Read the model definition and answer for the solid it produces. Units are mm, in the model's axes. A direction names the side the tool comes from. Coordinates: 2 decimals unless noted, no trailing zeros. Loops run counter-clockwise (first coordinate to the right, second up) from the corner with the lowest first, then second, coordinate; pieces in that order, holes last. Notation, with made-up numbers: M -32.5,1 L -12.5,1 A22 cw -12.5,21 Z; hole C 55.5,65 d4. An arc over 180 degrees is marked long. Use one line per item in the form item = value. Start each with the question number.
1. A tool of negligible diameter and unlimited length cuts with its end or side. For faces 4 (the flat face through (8.128, -19, 99)), 5 (the cylindrical face through (26.798, 52.192, 92.535)), from which of +Z, -Z, +X, -X, +Y, -Y can it reach the whole face along a straight path? Write none if from no direction.
2. The part is cut by section D-D (x = 4.5). Give the vertices of the cut face in (y, z), plus the area to 3 significant figures.
3. Find the intervals of material crossed by probe 1 along X at (y, z) = (-22, 98); probe 2 along Y at (x, z) = (21, 9); probe 3 along Z at (x, y) = (47, 33), in increasing order. Write a range as [from, to].
4. For a pull along X with two mould halves and no side action, classify faces 1 (the flat face through (46.228, -19, 99)), 2 (the flat face through (54.356, 10, 54)), 3 (the cylindrical face through (4.01, -15.1, 101.36)) as released by +X, released by -X, zero draft, split by the parting line, or undercut.
5. The part is cut by section A-A (x = 28.5). Give the vertices of the cut face in (y, z).
6. The part is cut by section B-B (z = 9). Give the vertices of the cut face in (x, y).
7. Flat-ended cylindrical pins translate along their axes: pin 1 (13 mm diameter, centred on y = -18, z = 102, fed in from -X); pin 2 (1 mm diameter, centred on x = 46, z = 40, fed in from +Y); pin 3 (12 mm diameter, centred on x = 44, y = 19, fed in from +Z); pin 4 (5 mm diameter, centred on x = 9.5, y = -18.5, fed in from +Z). Find the tip coordinate at first contact, or state that the pin passes through.
8. The part is cut by section C-C (y = 0.5). Give the vertices of the cut face in (x, z).
from build123d import *

# Parameters (mm, degrees)
F1_DEPTH = 54.356
F2_DEPTH = 8.128
F3_START = 38.1
F3_DEPTH = 8.128


with BuildPart() as f1:
    # F0 (on Right) → F1 (new body)
    with BuildSketch(Plane.YZ):
        with BuildLine():
            ThreePointArc((-15.3765147552, 0), (2.9971175827, 14.084579319), (21.3707499206, 0))
            Line((21.3707499206, 0), (36.0901206732, 0))
            Line((36.0901206732, 0), (46.1599725041, 83.5735037118))
            Line((46.1599725041, 83.5735037118), (47.4168173969, 94.0045341849))
            Line((47.4168173969, 94.0045341849), (-11.7700314149, 94.0045341849))
            Line((-11.7700314149, 94.0045341849), (-23.5962346196, 94.0045341849))
            Line((-23.5962346196, 94.0045341849), (-34.9229313433, 0))
            Line((-34.9229313433, 0), (-15.3765147552, 0))
        make_face()
        with BuildLine():
            Line((47.4168173969, 94.0045341849), (46.1599725041, 83.5735037118))
            ThreePointArc((46.1599725041, 83.5735037118), (51.9737480075, 83.9546377095), (55.2620962262, 88.7642130256))
            ThreePointArc((55.2620962262, 88.7642130256), (52.1340561486, 92.5739673663), (47.4168173969, 94.0045341849))
        make_face()
    extrude(amount=F1_DEPTH)

    # F0 (on Right) → F2 (join)
    with BuildSketch(Plane.YZ):
        with BuildLine():
            Line((-22.1934446874, 105.6468176636), (-23.5962346196, 94.0045341849))
            Line((-23.5962346196, 94.0045341849), (-11.7700314149, 94.0045341849))
            ThreePointArc((-11.7700314149, 94.0045341849), (-15.1754299061, 101.4428755336), (-22.1934446874, 105.6468176636))
        make_face()
    extrude(amount=F2_DEPTH)

    # F2_face (on face) → F3 (join)
    with BuildSketch(Plane(origin=(8.128, -18.3884037898, 98.5907501288), x_dir=(0, 1, 0), z_dir=(1, 0, 0)).offset(F3_START)):
        with BuildLine():
            ThreePointArc((6.6183723749, -4.5862159439), (3.2129738836, 2.8521254048), (-3.8050408977, 7.0560675348))
            Line((-3.8050408977, 7.0560675348), (-5.2078308298, -4.5862159439))
            Line((-5.2078308298, -4.5862159439), (6.6183723749, -4.5862159439))
        make_face()
    extrude(amount=F3_DEPTH)


solid = f1.part
Computed values:
q1.face_4 = +Z, +Y, -Y
q1.face_5 = +Z, +X, -X, +Y
q2.outline = M -34.92,0 L -15.38,0 A19.03 cw 21.37,0 L 36.09,0 L 46.16,83.57 A6.66 ccw 55.26,88.76 A8.49 ccw 47.42,94 L -11.77,94 A13.8 ccw -22.19,105.65 Z
q2.area = 6,460 mm²
q3.probe_1 = [0, 8.13], [46.23, 54.36]
q3.probe_2 = [-33.84, -9.95], [15.94, 37.17]
q3.probe_3 = [0, 94]
q4.face_1 = undercut
q4.face_2 = released by +X
q4.face_3 = zero draft
q5.outline = M -34.92,0 L -15.38,0 A19.03 cw 21.37,0 L 36.09,0 L 46.16,83.57 A6.66 ccw 55.26,88.76 A8.49 ccw 47.42,94 L -23.6,94 Z
q6.outline = M 0,-33.84 L 54.36,-33.84 L 54.36,-9.95 L 0,-9.95 Z; M 0,15.94 L 54.36,15.94 L 54.36,37.17 L 0,37.17 Z
q7.pin_1 = 0
q7.pin_2 = 40.97
q7.pin_3 = 94
q7.pin_4 = 105.15
q8.outline = M 0,13.92 L 54.36,13.92 L 54.36,94 L 0,94 Z
